Here's how the part is built. I have some questions about the finished solid (model axes, mm). A direction names the side the tool comes from. Round coordinates to 2 decimals unless told otherwise and drop trailing zeros. Order: outer loops, then holes, each group sorted by start corner. A loop starts at its lowest first (then second) coordinate and runs counter-clockwise, first axis right, second up. Notation, with made-up numbers: M 87,82 L 106,82 A16 ccw 106,102 Z; hole C 12,-25 d5. An arc over 180 degrees is marked long. Write item = value, one per line. Start each with the question number.
Item 1: I want a section at D-D, the plane x = 50.25. List the corners of the cut face in (y, z) for me.
Item 2: I'm going to push flat-ended pins straight in: P1, Ø1.4, axis at x = 47.5, y = 0.5, coming from the +Z side; P2, Ø0.6, axis at y = 0.5, z = 14.5, coming from the +X side. Where does each tip first touch, or does it pass through?
Item 3: I want a section at A-A, the plane y = 1.4. List the corners of the cut face in (x, z) for me.
Item 4: I want a section at C-C, the plane z = 13.4. List the corners of the cut face in (x, y) for me, plus the area to 3 significant figures.
Item 5: I want a section at B-B, the plane x = 48. List the corners of the cut face in (y, z) for me.
Item 6: For faces 1 (the face through (47, 1, 13.55)), 2 (the face through (49.43, 0.64, 13.81)), 3 (the face through (49.44, 0.64, 15.83)), which set-ups out of +Z, -Z, +X, -X, +Y, -Y let a thin tool reach every point of the face, with its end or its side?
Item 7: Please list where these lines run through material, in increasing order: L1, parallel to X at y = 0.25, z = 15.95; L2, parallel to Y at x = 50.75, z = 15.3; L3, parallel to Z at x = 46.25, y = 0.25.
```python
from build123d import *

# Parameters (mm, degrees)
EXTRUDE017_DEPTH = 1
EXTRUDE016_DEPTH = 2.25


with BuildPart() as extrude017:
    # Sketch017 → Extrude017 (new body)
    with BuildSketch(Plane.XZ):
        with BuildLine():
            ThreePointArc((11.7, 16.35), (11.063604, 16.086396), (10.8, 15.45))
            Line((10.8, 14.2), (10.8, 15.45))
            ThreePointArc((10.8, 14.2), (11.23934, 13.13934), (12.3, 12.7))
            Line((16.8, 12.7), (12.3, 12.7))
            ThreePointArc((16.8, 12.7), (17.86066, 13.13934), (18.3, 14.2))
            Line((18.3, 15.45), (18.3, 14.2))
            ThreePointArc((18.3, 15.45), (18.036396, 16.086396), (17.4, 16.35))
            Line((11.7, 16.35), (17.4, 16.35))
        make_face()
    extrude(amount=EXTRUDE017_DEPTH)


with BuildPart() as extrude017_1:
    # Extrude017 placement: moved
    add(extrude017.part.moved(Location((0, 2.5, 0))))


with BuildPart() as button002:
    # Sketch016 → Extrude016 (new body)
    with BuildSketch(Plane.XZ):
        with BuildLine():
            ThreePointArc((12.8, 16.1), (12.163604, 15.836396), (11.9, 15.2))
            Line((11.9, 14.45), (11.9, 15.2))
            ThreePointArc((11.9, 14.45), (12.163604, 13.813604), (12.8, 13.55))
            Line((16.3, 13.55), (12.8, 13.55))
            ThreePointArc((16.3, 13.55), (16.936396, 13.813604), (17.2, 14.45))
            Line((17.2, 15.2), (17.2, 14.45))
            ThreePointArc((17.2, 15.2), (16.936396, 15.836396), (16.3, 16.1))
            Line((12.8, 16.1), (16.3, 16.1))
        make_face()
    extrude(amount=EXTRUDE016_DEPTH)


with BuildPart() as button002_1:
    # Extrude016 placement: moved
    add(button002.part.moved(Location((0, 2, 0))))

    # Fusion021: union Extrude017
    add(extrude017_1.part)


with BuildPart() as button002_2:
    # Fusion021 placement: moved
    add(button002_1.part.moved(Location((32.5, 0, 0))))


solid = button002_2.part
```
Filled in:
q1.outline = M 1.5,13.04 L 2.5,13.04 L 2.5,16.28 L 1.5,16.28 Z
q2.P1 = 16.1
q2.P2 = 49.7
q3.outline = M 44.4,14.45 A0.9 ccw 45.3,13.55 L 48.8,13.55 A0.9 ccw 49.7,14.45 L 49.7,15.2 A0.9 ccw 48.8,16.1 L 45.3,16.1 A0.9 ccw 44.4,15.2 Z
q4.outline = M 43.53,1.5 L 50.57,1.5 L 50.57,2.5 L 43.53,2.5 Z
q4.area = 7.04 mm^2
q5.outline = M -0.25,13.55 L 1.5,13.55 L 1.5,12.7 L 2.5,12.7 L 2.5,16.35 L 1.5,16.35 L 1.5,16.1 L -0.25,16.1 Z
q6.face_1 = -Z, +X, -X, -Y
q6.face_2 = -Z, +X, -Y
q6.face_3 = +Z, +X, -Y
q7.L1 = 44.8 to 49.3
q7.L2 = 1.5 to 2.5
q7.L3 = 13.55 to 16.1
